Verification items for the finished model (mm, model axes). A direction names the side the tool comes from. Give positions to 0.01 mm unless a question says otherwise; leave off trailing zeros. Order: outer loops, then holes, each group sorted by start corner. A loop starts at its lowest first (then second) coordinate and runs counter-clockwise, first axis right, second up.
from build123d import *

# Parameters (mm, degrees)
F0_R      = 1.2
F0_W      = 31.75
F0_H      = 14.2875
F1_DEPTH  = 5
F2_W      = 19.05
F2_H      = 31.75
F3_DEPTH  = 5
F4_W      = 43.000006
F4_H      = 12.7
F5_DEPTH  = 5
F6_W      = 17.78
F6_H      = 17.78
F7_DEPTH  = 5
F8_W      = 12.610003
F8_H      = 12.7
F9_DEPTH  = 7.62
F10_R     = 3.175
F11_DEPTH = 7.62
F12_R     = 1.2
F13_DEPTH = 6
F14_W     = 3
F14_H     = 16.51
F15_DEPTH = 10
F16_R     = 1.349997
F17_DEPTH = 3


with BuildPart() as f1:
    # F0 (on Top) → F1 (new body)
    with BuildSketch(Plane.XY):
        Polygon((-31.75, 36.5125), (-12.7, 36.5125), (-12.7, 0), (0, 0), (0, 50.8), (-31.75, 50.8), align=None)
        with Locations((-26.9875, 39.84625)):
            Circle(F0_R, mode=Mode.SUBTRACT)
        with BuildLine():
            Line((0, 0), (-12.7, 0))
            Line((-12.7, 0), (-12.7, -36.5125))
            Line((-12.7, -36.5125), (-31.75, -36.5125))
            Line((-31.75, -36.5125), (-31.75, -50.8))
            Line((-31.75, -50.8), (0, -50.8))
            Line((0, -50.8), (0, -49.9875))
            ThreePointArc((0, -49.9875), (-2.6, -47.3875), (0, -44.7875))
            Line((0, -44.7875), (0, -37.2875))
            ThreePointArc((0, -37.2875), (-2.6, -34.6875), (0, -32.0875))
            Line((0, -32.0875), (0, -24.5875))
            ThreePointArc((0, -24.5875), (-2.6, -21.9875), (0, -19.3875))
            Line((0, -19.3875), (0, 0))
        make_face()
        with Locations((-26.9875, -39.84625)):
            Circle(F0_R, mode=Mode.SUBTRACT)
        with Locations((-10, -17.500003)):
            Circle(F0_R, mode=Mode.SUBTRACT)
        with Locations((-10, -7.499998)):
            Circle(F0_R, mode=Mode.SUBTRACT)
        Polygon((0, 50.8), (0, 0), (12.7, 0), (12.7, 36.5125), (31.75, 36.5125), (31.75, 50.8), align=None)
        with Locations((26.9875, 39.84625)):
            Circle(F0_R, mode=Mode.SUBTRACT)
        with BuildLine():
            Line((12.7, 0), (0, 0))
            Line((0, 0), (0, -19.3875))
            ThreePointArc((0, -19.3875), (1.838478, -20.149022), (2.6, -21.9875))
            ThreePointArc((2.6, -21.9875), (1.838478, -23.825978), (0, -24.5875))
            Line((0, -24.5875), (0, -32.0875))
            ThreePointArc((0, -32.0875), (1.838478, -32.849022), (2.6, -34.6875))
            ThreePointArc((2.6, -34.6875), (1.838478, -36.525978), (0, -37.2875))
            Line((0, -37.2875), (0, -44.7875))
            ThreePointArc((0, -44.7875), (1.838478, -45.549022), (2.6, -47.3875))
            ThreePointArc((2.6, -47.3875), (1.838478, -49.225978), (0, -49.9875))
            Line((0, -49.9875), (0, -50.8))
            Line((0, -50.8), (31.75, -50.8))
            Line((31.75, -50.8), (31.75, -36.5125))
            Line((31.75, -36.5125), (12.7, -36.5125))
            Line((12.7, -36.5125), (12.7, 0))
        make_face()
        with Locations((26.9875, -39.84625)):
            Circle(F0_R, mode=Mode.SUBTRACT)
        with Locations((10, -17.500003)):
            Circle(F0_R, mode=Mode.SUBTRACT)
        with Locations((10, -7.499998)):
            Circle(F0_R, mode=Mode.SUBTRACT)
        with Locations((-15.875, 57.94375)):
            Rectangle(F0_W, F0_H)
        with Locations((-26.9875, 61.75375)):
            Circle(F0_R, mode=Mode.SUBTRACT)
        with Locations((15.875, 57.94375)):
            Rectangle(F0_W, F0_H)
        with Locations((26.9875, 61.75375)):
            Circle(F0_R, mode=Mode.SUBTRACT)
        with BuildLine():
            Line((0, -50.8), (-31.75, -50.8))
            Line((-31.75, -50.8), (-31.75, -65.0875))
            Line((-31.75, -65.0875), (0, -65.0875))
            Line((0, -65.0875), (0, -62.6875))
            ThreePointArc((0, -62.6875), (-2.6, -60.0875), (0, -57.4875))
            Line((0, -57.4875), (0, -50.8))
        make_face()
        with Locations((-26.9875, -61.75375)):
            Circle(F0_R, mode=Mode.SUBTRACT)
        with BuildLine():
            Line((31.75, -50.8), (0, -50.8))
            Line((0, -50.8), (0, -57.4875))
            ThreePointArc((0, -57.4875), (1.838478, -58.249022), (2.6, -60.0875))
            ThreePointArc((2.6, -60.0875), (1.838478, -61.925978), (0, -62.6875))
            Line((0, -62.6875), (0, -65.0875))
            Line((0, -65.0875), (31.75, -65.0875))
            Line((31.75, -65.0875), (31.75, -50.8))
        make_face()
        with Locations((26.9875, -61.75375)):
            Circle(F0_R, mode=Mode.SUBTRACT)
    extrude(amount=F1_DEPTH)

    # F2 (on face) → F3 (join, through all)
    with BuildSketch(Plane.XY.offset(5)):
        with Locations((-22.225, 20.6375)):
            Rectangle(F2_W, F2_H)
        with Locations((22.225, 20.6375)):
            Rectangle(F2_W, F2_H)
    extrude(amount=-F3_DEPTH)

    # F4 (on face) → F5 (cut, through all)
    with BuildSketch(Plane.XY.offset(5)):
        with Locations((0, 58.7375)):
            Rectangle(F4_W, F4_H)
    extrude(amount=-F5_DEPTH, mode=Mode.SUBTRACT)

    # F6 (on face) → F7 (cut, through all)
    with BuildSketch(Plane(origin=(0, 0, 0), x_dir=(1, 0, 0), z_dir=(0, 0, -1))):
        with Locations((0, -43.4975)):
            Rectangle(F6_W, F6_H)
    extrude(amount=-F7_DEPTH, mode=Mode.SUBTRACT)

    # F8 (on face) → F9 (join)
    with BuildSketch(Plane.XY.offset(5)):
        with Locations((-15.195002, 46.0375)):
            Rectangle(F8_W, F8_H)
        with Locations((15.195002, 46.0375)):
            Rectangle(F8_W, F8_H)
    extrude(amount=F9_DEPTH)

    # F10 (on face) → F11 (cut)
    with BuildSketch(Plane.XY.offset(12.62)):
        with BuildLine():
            Line((-19.225006, 46.0375), (-12.875006, 46.0375))
            ThreePointArc((-12.875006, 46.0375), (-16.050006, 49.2125), (-19.225006, 46.0375))
        make_face()
        with BuildLine():
            ThreePointArc((-19.225006, 46.0375), (-16.050006, 42.8625), (-12.875006, 46.0375))
            Line((-12.875006, 46.0375), (-19.225006, 46.0375))
        make_face()
        with Locations((16.050006, 46.0375)):
            Circle(F10_R)
    extrude(amount=-F11_DEPTH, mode=Mode.SUBTRACT)

    # F12 (on face) → F13 (cut)
    with BuildSketch(Plane(origin=(0, 52.3875, 0), x_dir=(-1, 0, 0), z_dir=(0, 1, 0))):
        with Locations((17.500003, 8.81)):
            Circle(F12_R)
        with Locations((-17.500003, 8.81)):
            Circle(F12_R)
    extrude(amount=-F13_DEPTH, mode=Mode.SUBTRACT)

    # F14 (on face) → F15 (join)
    with BuildSketch(Plane.XY.offset(5)):
        with Locations((-30.25, 47.9425)):
            Rectangle(F14_W, F14_H)
    extrude(amount=F15_DEPTH)

    # F16 (on face) → F17 (cut, through all)
    with BuildSketch(Plane.YZ.offset(-28.75)):
        with Locations((42.917504, 11.599987)):
            Circle(F16_R)
        with Locations((52.967496, 11.599987)):
            Circle(F16_R)
    extrude(amount=-F17_DEPTH, mode=Mode.SUBTRACT)


solid = f1.part
(1) Section check A-A, the plane z = 8.81. Give the number of separate pieces and of enclosed holes in the cut face, then the cut area to 3 significant figures.
Solved:
separate pieces: 3
enclosed holes: 0
area: 289 mm2
(2) Release check for a two-part mould opening along X. For faces 6 (the flat face through (-12.7, -16, 2)), 7 (the cylindrical face through (25.79, -39.79, 2.46)), 8 (the cylindrical face through (-30.229, 41.846, 10.779)), 9 (the cylindrical face through (-27.144, -60.564, 2.465)) record: pulls with the +X half, pulls with the -X half, needs draft (parallel to the pull), parting line crosses it, or undercut.
Solved:
face 6: pulls with the -X half
face 7: undercut
face 8: needs draft
face 9: undercut
(3) Set-up check for faces 1 (the flat face through (-22, -36.512, 2)), 2 (the cylindrical face through (18.7, 50.63, 8.86)), 3 (the flat face through (-16, 46, 5)), 4 (the flat face through (0, 34.608, 2)), 5 (the flat face through (22, 4.762, 3)): record each of +Z, -Z, +X, -X, +Y, -Y from which the full face is reachable in a straight line by a thin tool's end or side.
Solved:
face 1: +Z, -Z, -X
face 2: +Y
face 3: +Z
face 4: +Z, -Z, +Y
face 5: +Z, -Z, +X
(4) Section check B-B, the plane y = 11.5. Enter the section's corners in (x, z), then the cut area to 4 significant figures.
Solved:
outline: (-31.75, 0) - (31.75, 0) - (31.75, 5) - (-31.75, 5) - close
area: 317.5 mm2
(5) Scan lines: line 1 (X direction, y = 50.75, z = 8.81); line 2 (Y direction, x = -16, z = 7.5); line 3 (Z direction, x = -1.5, y = 14). Record each from-to range of solid material in increasing order.
Solved:
line 1: x = -31.75 to -28.75, -21.5 to -18.7, -16.3 to -8.89, 8.89 to 16.3, 18.7 to 21.5
line 2: y = 39.69 to 42.86, 49.21 to 52.39
line 3: z = 0 to 5
(6) Go/stop test with flat-tipped pins: pin 1 (4 mm diameter, centred on y = -26, z = 3, fed in from -X); pin 2 (5.5 mm diameter, centred on x = -1, z = 1.5, fed in from +Y); pin 3 (6.5 mm diameter, centred on x = 12.5, z = 3, fed in from +Y); pin 4 (1.9 mm diameter, centred on x = -10, y = -7.5, fed in from +Z). Record where each tip stops, or that it passes through.
Solved:
pin 1: stops at x = -12.7
pin 2: stops at y = 34.61
pin 3: stops at y = 52.39
pin 4: passes through
